The drawing under review shows one solid part. Ordinate dimensions are in mm from its lowest x, y, z. A direction names the side the tool comes from. Coordinates: 2 decimals unless noted, no trailing zeros. Order: outer loops, then holes, each group sorted by start corner. A loop starts at its lowest first (then second) coordinate and runs counter-clockwise, first axis right, second up. Notation, with made-up numbers: (57, 23.25) - (104, 23.25) arc R18 ccw to (104, 44.25) - close; hole circle Ø5 at (36.25, 46). An arc over 180 degrees is marked (long way). Answer in a Markdown table with one row per item.
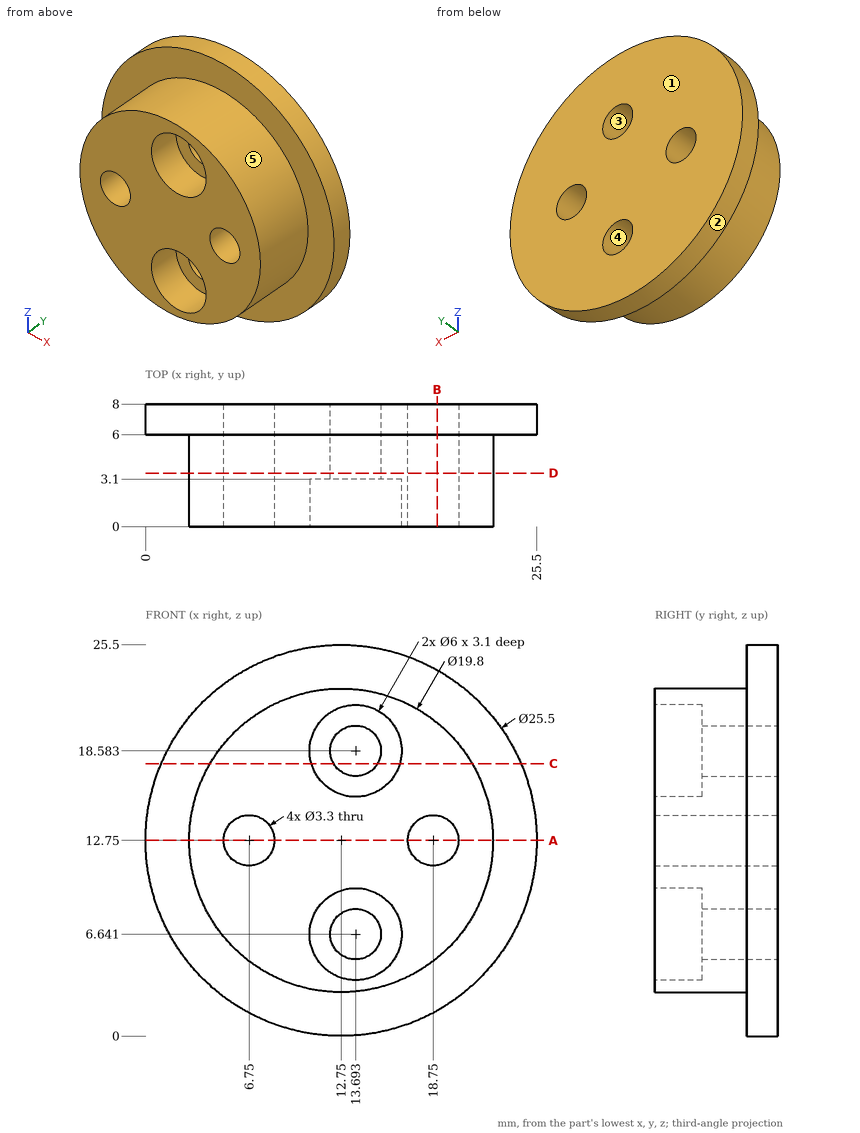
Item 1: We need section A-A, the plane z = 12.75. Write out the cut boundary in (x, y), then the cut area to 3 significant figures.
Check values:
| item | result |
|---|---|
| outline | (0, 6) - (2.85, 6) - (2.85, 0) - (5.1, 0) - (5.1, 8) - (0, 8) - close; (8.4, 0) - (17.1, 0) - (17.1, 8) - (8.4, 8) - close; (20.4, 0) - (22.65, 0) - (22.65, 6) - (25.5, 6) - (25.5, 8) - (20.4, 8) - close |
| area | 117 mm^2 |
Item 2: Clearance check with flat-ended pins moving along their axes: pin 1 Ø8 at (x, z) = (7, 13) entering from -Y; pin 2 Ø5 at (x, z) = (13.69, 18.58) entering from -Y; pin 3 Ø3 at (x, z) = (13.69, 18.58) entering from -Y; pin 4 Ø1.5 at (x, y) = (10, 2.5) entering from -Z. State where each tip first meets the part, or that it passes through.
Check values:
| item | result |
|---|---|
| pin 1 | y = 0 |
| pin 2 | y = 3.1 |
| pin 3 | through |
| pin 4 | z = 3.05 |
Item 3: We need section D-D, the plane y = 3.5. Write out the cut boundary in (x, z).
Check values:
| item | result |
|---|---|
| outline | circle Ø19.8 at (12.75, 12.75); hole circle Ø3.3 at (6.75, 12.75); hole circle Ø3.3 at (13.69, 6.64); hole circle Ø3.3 at (13.69, 18.58); hole circle Ø3.3 at (18.75, 12.75) |
Item 4: Mouldability with a two-part tool opening along Z and no side actions: class the marked faces 1, 2 and 3 as +Z half, -Z half, draft (parallel to the pull), parting line (faces both ways), or undercut.
Check values:
| item | result |
|---|---|
| face 1 | draft |
| face 2 | parting line |
| face 3 | undercut |
Item 5: We need section B-B, the plane x = 19. Write out the cut boundary in (y, z).
Check values:
| item | result |
|---|---|
| outline | (0, 5.07) - (6, 5.07) - (6, 1.64) - (8, 1.64) - (8, 11.12) - (0, 11.12) - close; (0, 14.38) - (8, 14.38) - (8, 23.86) - (6, 23.86) - (6, 20.43) - (0, 20.43) - close |
Item 6: To check wall thickness, follow line 1 (X direction, y = 5, z = 12.75); line 2 (X direction, y = 4.5, z = 12.25); line 3 (Z direction, x = 16, y = 2.75) (1 decimal). State the ranges of each line that lie inside material, in increasing order. Write a range as from..to.
Check values:
| item | result |
|---|---|
| line 1 | 2.85..5.1, 8.4..17.1, 20.4..22.65 |
| line 2 | 2.86..5.18, 8.32..17.18, 20.32..22.64 |
| line 3 | 3.4..4.7, 8.6..16.7, 20.5..22.1 |
Item 7: We need section C-C, the plane z = 17.75. Write out the cut boundary in (x, y) (1 decimal), then the cut area to 3 significant figures.
Check values:
| item | result |
|---|---|
| outline | (1, 6) - (4.2, 6) - (4.2, 0) - (10.8, 0) - (10.8, 3.1) - (12.3, 3.1) - (12.3, 8) - (1, 8) - close; (15.1, 3.1) - (16.6, 3.1) - (16.6, 0) - (21.3, 0) - (21.3, 6) - (24.5, 6) - (24.5, 8) - (15.1, 8) - close |
| area | 118 mm^2 |
Item 8: Tool access review of the marked faces 4 and 5: name each direction out of +Z, -Z, +X, -X, +Y, -Y from which nothing blocks a thin tool from reaching the whole face with its end or side.
Check values:
| item | result |
|---|---|
| face 4 | +Y, -Y |
| face 5 | -Y |
